The listing builds one solid part. Answer for the finished solid, in the listing's coordinates (mm). Face numbers are marked on the shaded views. A direction names the side the tool comes from. Round coordinates to 2 decimals unless told otherwise and drop trailing zeros. Loops run counter-clockwise (first coordinate to the right, second up) from the corner with the lowest first, then second, coordinate; pieces in that order, holes last. Notation, with made-up numbers: M 19,19 L 39,19 A13 ccw 39,23 Z; hole C 65.25,-24.75 d5. An arc over 180 degrees is marked long. Answer as a JSON object with one key per item and string values.
Solid Edge part; units mm, degrees
sketch "Sketch1" plane through (0, 0, 0) normal (0, 0, 1) x (1, 0, 0)
  line L0 (-105, 55) -> (-105, -55)
  line L1 (-105, -55) -> (105, -55)
  line L2 (105, -55) -> (105, 55)
  line L3 (105, 55) -> (-105, 55)
extrude "Protrusion1" add sketch "Sketch1" along normal blind 8
sketch "Sketch2" plane through (0, 0, 0) normal (0, 0, -1) x (1, 0, 0)
  line L0 (-94.0409, -50.5) -> (94.0409, -50.5)
  arc A0 (95.9257, -51.3576) -> (94.0409, -50.5) centre (94.0409, -53) ccw
  arc A1 (101.3576, -45.9257) -> (95.9257, -51.3576) centre (98.8284, -48.8284) cw
  arc A2 (100.5, -44.0409) -> (101.3576, -45.9257) centre (103, -44.0409) ccw
  line L1 (100.5, -44.0409) -> (100.5, 44.0409)
  arc A3 (101.3576, 45.9257) -> (100.5, 44.0409) centre (103, 44.0409) ccw
  arc A4 (95.9359, 51.3692) -> (101.3576, 45.9257) centre (98.8284, 48.8284) cw
  arc A5 (94.0579, 50.5191) -> (95.9359, 51.3692) centre (94.0576, 53.0191) ccw
  line L2 (94.0579, 50.5191) -> (-94.0408, 50.5001)
  arc A6 (-95.9258, 51.3577) -> (-94.0408, 50.5001) centre (-94.041, 53.0001) ccw
  arc A7 (-101.3576, 45.9257) -> (-95.9258, 51.3577) centre (-98.8284, 48.8284) cw
  arc A8 (-100.5, 44.0409) -> (-101.3576, 45.9257) centre (-103, 44.0409) ccw
  line L3 (-100.5, 44.0409) -> (-100.5, -44.0409)
  arc A9 (-101.3576, -45.9257) -> (-100.5, -44.0409) centre (-103, -44.0409) ccw
  arc A10 (-95.9257, -51.3576) -> (-101.3576, -45.9257) centre (-98.8284, -48.8284) cw
  arc A11 (-94.0409, -50.5) -> (-95.9257, -51.3576) centre (-94.0409, -53) ccw
  line L4 (97, -43) -> (97, 43)
  arc A12 (93, 47) -> (97, 43) centre (93, 43) cw
  line L5 (93, 47) -> (-93, 47)
  arc A13 (-97, 43) -> (-93, 47) centre (-93, 43) cw
  line L6 (-97, 43) -> (-97, -43)
  arc A14 (-97, -43) -> (-93, -47) centre (-93, -43) ccw
  line L7 (-93, -47) -> (93, -47)
  arc A15 (97, -43) -> (93, -47) centre (93, -43) cw
extrude "Wycięcie_1" cut sketch "Sketch2" against normal blind 6.5
sketch "Sketch3" plane through (0, 0, 0) normal (0, 0, -1) x (1, 0, 0)
  circle A0 centre (-98.8284, 48.8284) radius 1.5
  circle A1 centre (98.8284, 48.8284) radius 1.5
  circle A2 centre (98.8284, -48.8284) radius 1.5
  circle A3 centre (-98.8284, -48.8284) radius 1.5
extrude "Wycięcie_2" cut sketch "Sketch3" against normal blind 159.0153
fillet "Zaokrąglenie_1" radius 4 4 edges at (105, -55, 4) (105, 55, 4) (-105, 55, 4) (-105, -55, 4)
sketch "Sketch4" plane through (0, 0, 8) normal (0, 0, 1) x (0, 1, 0)
  line L0 (55, -61) -> (75, -61)
  line L1 (75, -61) -> (75, -91)
  line L2 (75, -91) -> (55, -91)
  line L3 (50.5, -91) -> (55, -91)
  line L4 (50.5, -61) -> (50.5, -91)
  line L5 (55, -61) -> (50.5, -61)
  line L6 (-32.0409, -125) -> (-32.0409, -105)
  line L7 (-32.0409, -105) -> (-32.0409, -100.5)
  line L8 (-32.0409, -100.5) -> (-2.0409, -100.5)
  line L9 (-2.0409, -100.5) -> (-2.0409, -105)
  line L10 (-2.0409, -105) -> (-2.0409, -125)
  line L11 (-2.0409, -125) -> (-32.0409, -125)
extrude "Wyciągnięcie_2" add sketch "Sketch4" against normal blind 45
sketch "Sketch5" plane through (76, 65, -37) normal (0, 0, -1) x (-1, 0, 0)
  line L0 (-12.5, -15.515) -> (12.5, -15.515)
  line L1 (12.5, -15.515) -> (12.5, 7.5)
  line L2 (0, 7.5) -> (12.5, 7.5)
  line L3 (0, 7.5) -> (-12.5, 7.5)
  line L4 (-12.5, 7.5) -> (-12.5, -15.515)
  line L5 (-46.5, -82.0409) -> (-46.5, -69.5409)
  line L6 (-46.5, -69.5409) -> (-23.2142, -69.5409)
  line L7 (-23.2142, -69.5409) -> (-23.2142, -94.5409)
  line L8 (-23.2142, -94.5409) -> (-46.5, -94.5409)
  line L9 (-46.5, -94.5409) -> (-46.5, -82.0409)
extrude "Wycięcie_3" cut sketch "Sketch5" against normal blind 36
fillet "Zaokrąglenie_2" radius 5 12 edges at (105, -2.0409, 4) (125, -2.0409, -14.5) (125, -32.0409, -14.5) (105, -32.0409, 4) (91, 75, -14.5) (91, 55, 4) (61, 55, 4) (61, 75, -14.5) (63.5, 72.5, -19) (88.5, 72.5, -19) (122.5, -4.5409, -19) (122.5, -29.5409, -19)
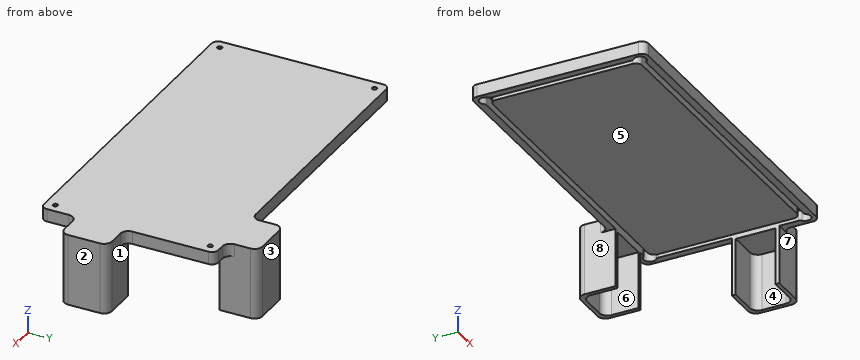
Item 1: The part is cut by section B-B (y = -12.5). Give the vertices of the cut face in (x, z), then the cut area to 3 significant figures.
Values follow:
{"outline": "M -105,0 L -100.5,0 L -100.5,6.5 L -97,6.5 L -97,0 L 97,0 L 97,6.5 L 100.5,6.5 L 100.5,-1 L 122.5,-1 L 122.5,-37 L 125,-37 L 125,8 L -105,8 Z", "area": "1,910 mm^2"}
Item 2: The part is cut by section C-C (x = -82). Give the vertices of the cut face in (y, z), then the cut area to 3 significant figures.
Values follow:
{"outline": "M -55,0 L -50.5,0 L -50.5,6.5 L -47,6.5 L -47,0 L 47,0 L 47,6.5 L 50.5,6.5 L 50.5,0 L 55,0 L 55,8 L -55,8 Z", "area": "834 mm^2"}
Item 3: Flat-ended cylindrical pins translate along their axes: P1, Ø21.5, axis at x = 109, z = -7.5, coming from the +Y side; P2, Ø12, axis at x = 71, z = -25.5, coming from the -Y side; P3, Ø15, axis at x = 101.5, y = 41, coming from the -Z side; P4, Ø10, axis at y = -37.5, z = -9.5, coming from the +X side. Find the tip coordinate at first contact, or state that the pin passes through.
Values follow:
{"P1": "y = 54.99", "P2": "y = 71.07", "P3": "z = 0", "P4": "through"}
Item 4: Which of the six approach directions +Z, -Z, +X, -X, +Y, -Y give full straight-line access (tool end or side, diameter ignored) to the marked faces 1, 2, 3, 4 and 5?
Values follow:
{"face 1": "-Z, +X, +Y", "face 2": "+Z, -Z, +X, +Y, -Y", "face 3": "+Z, -Z, +X, -X, +Y", "face 4": "-Z, -X", "face 5": "-Z, -X, -Y"}
Item 5: Determine the mould class of the marked faces 6, 7 and 8 for opening direction X: released by +X, released by -X, zero draft, split by the parting line, or undercut.
Values follow:
{"face 6": "undercut", "face 7": "zero draft", "face 8": "released by -X"}
Item 6: Straight lines are drawn through the part: line 1 (X direction, y = 8, z = 4); line 2 (Y direction, x = -28.5, z = 5); line 3 (Y direction, x = 114, z = -15.5). For each, find the intervals that lie inside material, in ascending order.
Values follow:
{"line 1": "-105 to -100.5, -97 to 97, 100.5 to 105", "line 2": "-55 to -50.51, -47 to 47, 50.5 to 55", "line 3": "-32.04 to -29.54, -4.54 to -2.04"}
Item 7: The part is cut by section D-D (y = 40). Give the vertices of the cut face in (x, z).
Values follow:
{"outline": "M -105,0 L -100.5,0 L -100.5,6.5 L -97,6.5 L -97,0 L 97,0 L 97,6.5 L 100.5,6.5 L 100.5,0 L 105,0 L 105,8 L -105,8 Z"}
Item 8: The part is cut by section A-A (z = -33). Give the vertices of the cut face in (x, y), then the cut area to 3 significant figures.
Values follow:
{"outline": "M 61,50.5 L 63.5,50.5 L 63.5,67.5 A5 cw 68.5,72.5 L 83.5,72.5 A5 cw 88.5,67.5 L 88.5,50.5 L 91,50.5 L 91,70 A5 ccw 86,75 L 66,75 A5 ccw 61,70 Z; M 100.5,-32.04 L 120,-32.04 A5 ccw 125,-27.04 L 125,-7.04 A5 ccw 120,-2.04 L 100.5,-2.04 L 100.5,-4.54 L 117.5,-4.54 A5 cw 122.5,-9.54 L 122.5,-24.54 A5 cw 117.5,-29.54 L 100.5,-29.54 Z", "area": "370 mm^2"}
